Design review of the part built by this model. Coordinates are the model's own, in mm. A direction names the side the tool comes from. Give positions to 0.01 mm unless a question says otherwise; leave off trailing zeros. Loops run counter-clockwise (first coordinate to the right, second up) from the corner with the lowest first, then second, coordinate; pieces in that order, holes last. Notation, with made-up numbers: (44, -21.75) - (91, -21.75) arc R22 ccw to (91, -10.75) - close; hole circle Ø4 at (35, -37). An arc over 180 degrees is marked (long way). Write each question's results on one line, items separated by ' | '.
```python
from build123d import *

# Parameters (mm, degrees)
EXTRUDE_1_DEPTH          = 3
PATTERN_LINEAR_2_COUNT   = 2
PATTERN_LINEAR_2_PITCH   = 23
EXTRUDE_2_DEPTH          = 26
SKETCH_3_R               = 1.85
CUT_EXTRUDE_1_DEPTH      = 10
CUT_EXTRUDE_2_DEPTH      = 24
CUT_EXTRUDE_START        = -2.5
SKETCH_5_W               = 4
SKETCH_5_H               = 10
CUT_EXTRUDE_3_DEPTH      = 2.5
FILLET_3_R               = 2
EXTRUDE_START            = -10
SKETCH_7_W               = 9.83
SKETCH_7_H               = 10
SKETCH_7_W_2             = 10
EXTRUDE_4_DEPTH          = 5.55
CUT_EXTRUDE_4_REACH      = 21.469
SKETCH_8_R               = 1.5
SKETCH_10_W              = 15
SKETCH_10_H              = 21.87
CUT_EXTRUDE_5_DEPTH      = 37
CUT_EXTRUDE_6_DEPTH      = 11
CUT_EXTRUDE_6_DEPTH_BACK = 37
SKETCH_12_R              = 1.85
EXTRUDE_5_DEPTH          = 2.4
SKETCH_13_W              = 10.554856858
SKETCH_13_H              = 20
CUT_EXTRUDE_7_DEPTH      = 3.419156865
SKETCH_14_W              = 41.2
SKETCH_14_H              = 20.3
CUT_EXTRUDE_8_DEPTH      = 32.719156865


with BuildPart() as part:
    # Sketch 1 → Extrude 1 (new body)
    with BuildSketch(Plane(origin=(0, 0, 0), x_dir=(1, 0, 0), z_dir=(0, 1, 0))):
        with BuildLine():
            Line((-47.15, 10.148849956), (-17.708435007, 10.148849956))
            ThreePointArc((-17.708435007, 10.148849956), (-17.806599121, 9.727806242), (-17.973176083, 9.328849956))
            ThreePointArc((-17.973176083, 9.328849956), (-20.25, 0), (-17.973176083, -9.328849956))
            ThreePointArc((-17.973176083, -9.328849956), (-17.79606457, -11.292053253), (-19.04716249, -12.815302961))
            ThreePointArc((-19.04716249, -12.815302961), (-19.687557209, -13.232647403), (-20.25, -13.750276505))
            Line((-20.25, -13.750276505), (-20.25, -30.751150044))
            Line((-20.25, -30.751150044), (-47.15, -30.751150044))
            Line((-47.15, -30.751150044), (-47.15, 10.148849956))
        make_face()
    extrude(amount=EXTRUDE_1_DEPTH)


with BuildPart() as pattern_linear_2_1:
    # Pattern Linear 2: pattern copy
    add(part.part.moved(Location(Vector(0, 1, 0) * (1 * PATTERN_LINEAR_2_PITCH))))


with BuildPart() as part_1:
    add(part.part)

    add(pattern_linear_2_1.part)  # Extrude 2 merges Pattern Linear 2_1
    # Sketch 2 → Extrude 2 (add, through all)
    with BuildSketch(Plane(origin=(0, 26, 0), x_dir=(1, 0, 0), z_dir=(0, 1, 0))):
        with BuildLine():
            ThreePointArc((-18.778786242, 12.648849956), (-17.890693286, 11.549948159), (-17.708435007, 10.148849956))
            Line((-17.708435007, 10.148849956), (-47.15, 10.148849956))
            Line((-47.15, 10.148849956), (-47.15, 19.438849956))
            Line((-47.15, 19.438849956), (-35.15, 19.438849956))
            Line((-35.15, 19.438849956), (-35.15, 12.648849956))
            Line((-35.15, 12.648849956), (-18.778786242, 12.648849956))
        make_face()
        with BuildLine():
            Line((-20.25, -19.978716958), (-20.25, -30.751150044))
            Line((-20.25, -30.751150044), (-47.15, -30.751150044))
            Line((-47.15, -30.751150044), (-47.15, -40.041150044))
            Line((-47.15, -40.041150044), (-35.15, -40.041150044))
            Line((-35.15, -40.041150044), (-35.15, -33.251150044))
            Line((-35.15, -33.251150044), (-17.75, -33.251150044))
            Line((-17.75, -33.251150044), (-17.75, -21.378462168))
            ThreePointArc((-17.75, -21.378462168), (-19.111760818, -20.878198779), (-20.25, -19.978716958))
        make_face()
    extrude(amount=-EXTRUDE_2_DEPTH)

    # Sketch 3 → Cut-Extrude 1 (cut)
    with BuildSketch(Plane.ZY.offset(47.15)):
        with Locations((-13.948849956, 8)):
            Circle(SKETCH_3_R)
        with Locations((-13.948849956, 18)):
            Circle(SKETCH_3_R)
        with Locations((34.551150044, 18)):
            Circle(SKETCH_3_R)
        with Locations((34.551150044, 8)):
            Circle(SKETCH_3_R)
    extrude(amount=-CUT_EXTRUDE_1_DEPTH, mode=Mode.SUBTRACT)

    # Sketch 4 → Cut-Extrude 2 (cut)
    with BuildSketch(Plane.ZY.offset(47.15)):
        Polygon((-10.148849956, 15.5), (-12.648849956, 15.5), (-12.648849956, 14.5), (-14.148849956, 14.5), (-14.148849956, 11.5), (-12.648849956, 11.5), (-12.648849956, 10.5), (-10.148849956, 10.5), align=None)
    extrude(amount=-CUT_EXTRUDE_2_DEPTH, mode=Mode.SUBTRACT)

    # Sketch 5 → Cut-Extrude 3 (cut)
    with BuildSketch(Plane(origin=(0, 0, -12.648849956), x_dir=(-1, 0, 0), z_dir=(0, 0, -1)).offset(CUT_EXTRUDE_START)):
        with Locations((25.15, 13)):
            Rectangle(SKETCH_5_W, SKETCH_5_H)
    extrude(amount=CUT_EXTRUDE_3_DEPTH, mode=Mode.SUBTRACT)

    # Fillet 3
    fillet_3_edges = [part_1.edges().sort_by_distance(p)[0] for p in [
        (-41.15, 26, -19.438849956),
        (-41.15, 0, -19.438849956),
        (-41.15, 0, 40.041150044),
        (-41.15, 26, 40.041150044),
    ]]
    fillet(fillet_3_edges, radius=FILLET_3_R)

    # Sketch 7 → Extrude 4 (add)
    with BuildSketch(Plane.ZY.offset(47.15).offset(EXTRUDE_START)):
        with Locations((-7.733849956, 31)):
            Rectangle(SKETCH_7_W, SKETCH_7_H)
        with Locations((24.051150044, 31)):
            Rectangle(SKETCH_7_W_2, SKETCH_7_H)
        with Locations((-7.733849956, -5)):
            Rectangle(SKETCH_7_W, SKETCH_7_H)
        with Locations((24.051150044, -5)):
            Rectangle(SKETCH_7_W_2, SKETCH_7_H)
    extrude(amount=-EXTRUDE_4_DEPTH)

    # Sketch 8 → Cut-Extrude 4 (cut, up to next)
    with BuildSketch(Plane.ZY.offset(37.15), mode=Mode.PRIVATE) as cut_extrude_4_sk1:
        with Locations((-7.818849956, -5)):
            Circle(SKETCH_8_R)
    cut_extrude_4_tool1 = extrude(cut_extrude_4_sk1.sketch, amount=-CUT_EXTRUDE_4_REACH, mode=Mode.PRIVATE) & part_1.part
    add(cut_extrude_4_tool1.solids().sort_by_distance((-37.15, -5, -7.81885))[0], mode=Mode.SUBTRACT)
    # Sketch 8 → Cut-Extrude 4 (cut, up to next)
    with BuildSketch(Plane.ZY.offset(37.15), mode=Mode.PRIVATE) as cut_extrude_4_sk2:
        with Locations((-7.818849956, 31)):
            Circle(SKETCH_8_R)
    cut_extrude_4_tool2 = extrude(cut_extrude_4_sk2.sketch, amount=-CUT_EXTRUDE_4_REACH, mode=Mode.PRIVATE) & part_1.part
    add(cut_extrude_4_tool2.solids().sort_by_distance((-37.15, 31, -7.81885))[0], mode=Mode.SUBTRACT)
    # Sketch 8 → Cut-Extrude 4 (cut, up to next)
    with BuildSketch(Plane.ZY.offset(37.15), mode=Mode.PRIVATE) as cut_extrude_4_sk3:
        with Locations((24.051150044, 31)):
            Circle(SKETCH_8_R)
    cut_extrude_4_tool3 = extrude(cut_extrude_4_sk3.sketch, amount=-CUT_EXTRUDE_4_REACH, mode=Mode.PRIVATE) & part_1.part
    add(cut_extrude_4_tool3.solids().sort_by_distance((-37.15, 31, 24.05115))[0], mode=Mode.SUBTRACT)
    # Sketch 8 → Cut-Extrude 4 (cut, up to next)
    with BuildSketch(Plane.ZY.offset(37.15), mode=Mode.PRIVATE) as cut_extrude_4_sk4:
        with Locations((24.051150044, -5)):
            Circle(SKETCH_8_R)
    cut_extrude_4_tool4 = extrude(cut_extrude_4_sk4.sketch, amount=-CUT_EXTRUDE_4_REACH, mode=Mode.PRIVATE) & part_1.part
    add(cut_extrude_4_tool4.solids().sort_by_distance((-37.15, -5, 24.05115))[0], mode=Mode.SUBTRACT)

    # Sketch 10 → Cut-Extrude 5 (cut, through all)
    with BuildSketch(Plane.XZ):
        with Locations((-34.65, 8.116150044)):
            Rectangle(SKETCH_10_W, SKETCH_10_H)
    extrude(amount=-CUT_EXTRUDE_5_DEPTH, mode=Mode.SUBTRACT)

    # Sketch 11 → Cut-Extrude 6 (cut, two sides)
    with BuildSketch(Plane(origin=(0, 26, 0), x_dir=(1, 0, 0), z_dir=(0, 1, 0))) as cut_extrude_6_sk:
        with BuildLine():
            Line((-17.75, -33.251150044), (-17.75, -21.378462168))
            ThreePointArc((-17.75, -21.378462168), (-19.111760818, -20.878198779), (-20.25, -19.978716958))
            Line((-20.25, -19.978716958), (-20.25, -13.750276505))
            ThreePointArc((-20.25, -13.750276505), (-19.687557209, -13.232647403), (-19.04716249, -12.815302961))
            ThreePointArc((-19.04716249, -12.815302961), (-17.79606457, -11.292053253), (-17.973176083, -9.328849956))
            ThreePointArc((-17.973176083, -9.328849956), (-20.25, 0), (-17.973176083, 9.328849956))
            ThreePointArc((-17.973176083, 9.328849956), (-17.754165646, 11.139735768), (-18.778786242, 12.648849956))
            Line((-18.778786242, 12.648849956), (-18.928786242, 12.648849956))
            Line((-18.928786242, 12.648849956), (-18.928786242, 12.569773384))
            ThreePointArc((-18.928786242, 12.569773384), (-17.909278274, 11.141591723), (-18.10631072, 9.397952548))
            ThreePointArc((-18.10631072, 9.397952548), (-20.4, 0), (-18.10631072, -9.397952548))
            ThreePointArc((-18.10631072, -9.397952548), (-17.939417179, -11.247894117), (-19.118336373, -12.683264034))
            ThreePointArc((-19.118336373, -12.683264034), (-19.80280754, -13.132362008), (-20.4, -13.6923182))
            Line((-20.4, -13.6923182), (-20.4, -20.036675263))
            ThreePointArc((-20.4, -20.036675263), (-19.264296699, -20.963699107), (-17.9, -21.500252655))
            Line((-17.9, -21.500252655), (-17.9, -33.251150044))
            Line((-17.9, -33.251150044), (-17.75, -33.251150044))
        make_face()
    extrude(amount=CUT_EXTRUDE_6_DEPTH, mode=Mode.SUBTRACT)
    extrude(cut_extrude_6_sk.sketch, amount=-CUT_EXTRUDE_6_DEPTH_BACK, mode=Mode.SUBTRACT)

    # Sketch 12 → Extrude 5 (add)
    with BuildSketch(Plane.ZY.offset(47.15)):
        with BuildLine():
            Line((-17.438849956, 26), (38.041150044, 26))
            ThreePointArc((38.041150044, 26), (39.455363607, 25.414213562), (40.041150044, 24))
            Line((40.041150044, 24), (40.041150044, 2))
            ThreePointArc((40.041150044, 2), (39.455363607, 0.585786438), (38.041150044, 0))
            Line((38.041150044, 0), (-17.438849956, 0))
            ThreePointArc((-17.438849956, 0), (-18.853063518, 0.585786438), (-19.438849956, 2))
            Line((-19.438849956, 2), (-19.438849956, 24))
            ThreePointArc((-19.438849956, 24), (-18.853063518, 25.414213562), (-17.438849956, 26))
        make_face()
        with Locations((34.551150044, 18)):
            Circle(SKETCH_12_R, mode=Mode.SUBTRACT)
        with Locations((-13.948849956, 18)):
            Circle(SKETCH_12_R, mode=Mode.SUBTRACT)
        with Locations((-13.948849956, 8)):
            Circle(SKETCH_12_R, mode=Mode.SUBTRACT)
        with Locations((34.551150044, 8)):
            Circle(SKETCH_12_R, mode=Mode.SUBTRACT)
        Polygon((-10.148849956, 23), (-10.148849956, 15.5), (-12.648849956, 15.5), (-12.648849956, 14.5), (-14.148849956, 14.5), (-14.148849956, 11.5), (-12.648849956, 11.5), (-12.648849956, 10.5), (-10.148849956, 10.5), (-10.148849956, 3), (30.751150044, 3), (30.751150044, 23), align=None, mode=Mode.SUBTRACT)
    extrude(amount=EXTRUDE_5_DEPTH)

    # Sketch 13 → Cut-Extrude 7 (cut, through all)
    with BuildSketch(Plane.ZY.offset(20.25)):
        with Locations((25.473721615, 13)):
            Rectangle(SKETCH_13_W, SKETCH_13_H)
    extrude(amount=-CUT_EXTRUDE_7_DEPTH, mode=Mode.SUBTRACT)

    # Sketch 14 → Cut-Extrude 8 (cut, through all)
    with BuildSketch(Plane.ZY.offset(49.55)):
        with Locations((10.301150044, 13)):
            Rectangle(SKETCH_14_W, SKETCH_14_H)
    extrude(amount=-CUT_EXTRUDE_8_DEPTH, mode=Mode.SUBTRACT)


solid = part_1.part
```
Item 1: We need section D-D on x = -30.5. Give the boundary of the cut face in (y, z), then the cut area to 3 significant figures.
Output values:
outline: (0, -12.65) - (10.5, -12.65) - (10.5, -10.3) - (2.85, -10.3) - (2.85, -2.82) - (0, -2.82) - close; (0, 19.05) - (2.85, 19.05) - (2.85, 30.9) - (23.15, 30.9) - (23.15, 19.05) - (26, 19.05) - (26, 33.25) - (0, 33.25) - close; (15.5, -12.65) - (26, -12.65) - (26, -2.82) - (23.15, -2.82) - (23.15, -10.3) - (15.5, -10.3) - close | area: 221 mm²
Item 2: Clearance check with flat-ended pins moving along their axes: P1, Ø6, axis at y = 8, z = 34.55, coming from the +X side; P2, Ø1.5, axis at x = -33, y = 22, coming from the +Z side; P3, Ø2, axis at y = -2.5, z = 20, coming from the +X side; P4, Ø3, axis at x = -40.5, z = 1.5, coming from the -Y side. State where each tip first meets the part, or that it passes through.
Output values:
P1: stops at x = -17.9 | P2: stops at z = 33.25 | P3: stops at x = -31.6 | P4: passes through
Item 3: Draft analysis for pull direction Z (two halves, no side actions). For faces 1 (the face through (-49.55, 2, 11)), 2 (the face through (-34, -5, 29.051)), 3 (the face through (-19.282, 24.595, 20.953)), state which applies: +Z half, -Z half, draft (parallel to the pull), parting line (faces both ways), or undercut.
Output values:
face 1: draft | face 2: +Z half | face 3: undercut
Item 4: Tool access review of faces 4 (the face through (-37.15, 8, -14)), 5 (the face through (-26.9, 23.15, 10)), 6 (the face through (-31.6, -5, -6)), 7 (the face through (-35.15, 13, -16)): name each direction out of +Z, -Z, +X, -X, +Y, -Y from which nothing blocks a thin tool from reaching the whole face with its end or side.
Output values:
face 4: -X | face 5: +X, -X | face 6: +Z, -Z, +X, -Y | face 7: -Z, +X, +Y, -Y
Item 5: We need section B-B on y = -2.5. Give the boundary of the cut face in (x, z), then the cut area to 3 significant figures.
Output values:
outline: (-37.15, -12.65) - (-31.6, -12.65) - (-31.6, -2.82) - (-37.15, -2.82) - close; (-37.15, 19.05) - (-31.6, 19.05) - (-31.6, 29.05) - (-37.15, 29.05) - close | area: 110 mm²
Item 6: Wall thickness on probe 1 along Y at (x, z) = (-46, 15); probe 2 along Z at (x, y) = (-44, 23): over which ranges is each line inside the solid? List them lowest first.
Output values:
probe 1: y = 0 to 2.85, 23.15 to 26 | probe 2: z = -19.44 to -10.3, 30.9 to 40.04
Item 7: We need section A-A on x = -34. Give the boundary of the cut face in (y, z), then the cut area to 3 significant figures.
Output values:
outline: (-10, -12.65) - (10.5, -12.65) - (10.5, -10.3) - (2.85, -10.3) - (2.85, -2.82) - (-10, -2.82) - close; (-10, 19.05) - (2.85, 19.05) - (2.85, 30.9) - (23.15, 30.9) - (23.15, 19.05) - (36, 19.05) - (36, 29.05) - (26, 29.05) - (26, 33.25) - (0, 33.25) - (0, 29.05) - (-10, 29.05) - close; (15.5, -12.65) - (36, -12.65) - (36, -2.82) - (23.15, -2.82) - (23.15, -10.3) - (15.5, -10.3) - close; hole circle Ø3 at (-5, -7.82); hole circle Ø3 at (-5, 24.05); hole circle Ø3 at (31, -7.82); hole circle Ø3 at (31, 24.05) | area: 589 mm²
Item 8: We need section C-C on z = 0. Give the boundary of the cut face in (x, y).
Output values:
outline: (-49.55, 0) - (-42.15, 0) - (-42.15, 2.85) - (-49.55, 2.85) - close; (-49.55, 23.15) - (-42.15, 23.15) - (-42.15, 26) - (-49.55, 26) - close; (-27.15, 0) - (-20.4, 0) - (-20.4, 2.85) - (-27.15, 2.85) - close; (-27.15, 23.15) - (-20.4, 23.15) - (-20.4, 26) - (-27.15, 26) - close
